Here's how the part is built. I have some questions about the finished solid (model axes, mm). A direction names the side the tool comes from. Give positions to 0.01 mm unless a question says otherwise; leave off trailing zeros. Write each loop counter-clockwise with the first axis right and the second up, starting at its lowest first coordinate (ties: lowest second). Pieces come first, ordered by that corner, then holes. Notation, with made-up numbers: (30.25, -38) -> (75.25, -38) arc R19 ccw to (75.25, -29) -> close; hole circle Ø11 at (-37.5, 55). An arc over 180 degrees is marked (long way). Return JSON: item names as keys, results as strings.
Solid Edge part; units mm, degrees
sketch "Sketch1" plane through (0, 0, 0) normal (0, -1, 0) x (1, 0, 0)
  line L0 (-10, -30.5) -> (0, -30.5)
  line L1 (0, 30.5) -> (0, -30.5)
  line L2 (0, 30.5) -> (-10, 30.5)
  line L3 (-10, 30.5) -> (-10, -30.5)
revolve "RevolvedProtrusion1" add sketch "Sketch1" angle 360 about axis through (0, 0, 54) along (0, 0, -1)
sketch "Sketch2" plane through (0, 0, 0) normal (1, 0, 0) x (0, 1, 0)
  circle A0 centre (0, 2) radius 10
extrude "Protrusion1" add sketch "Sketch2" along normal blind 150
sketch "Sketch3" plane through (0, 0, 0) normal (0, 0, 1) x (1, 0, 0)
  circle A0 centre (-25.6627, -96.6511) radius 5
  line L0 (-8.9463, -4.4682) -> (-32.9115, -94.7264)
  arc A1 (-32.9115, -94.7264) -> (-18.4138, -98.5758) centre (-25.6627, -96.6511) ccw
  line L1 (-18.4138, -98.5758) -> (5.5514, -8.3176)
  arc A2 (5.5514, -8.3176) -> (-8.9463, -4.4682) centre (0, 0) cw
  dimension "D1" = 32.9115
  dimension "D2" = 25.6627
extrude "Styrarm" add sketch "Sketch3" along normal mid plane 10
hole "Hole1" at (0, 0, 30.5) direction (0, 0, -1) diameter 10 end up to next
1. For pin 1 Ø5 at (x, z) = (46, 11.5) entering from -Y; pin 2 Ø1.5 at (x, z) = (67, 6) entering from +Y; pin 3 Ø10 at (y, z) = (-8, 2) entering from -X, each with a flat end and sliding along its axis, tell me the tip position at first contact or that it passes through.
Taken from the geometry:
{"pin 1": "stops at y = -7.14", "pin 2": "stops at y = 9.46", "pin 3": "stops at x = -11.21"}
2. Suppose I cut it at D-D, the plane x = 99. List the corners of the cut face in (y, z) for me.
Taken from the geometry:
{"outline": "circle Ø20 at (0, 2)"}
3. Suppose I cut it at B-B, the plane z = 2. List the corners of the cut face in (x, y) for me, and give its area (3 significant figures).
Taken from the geometry:
{"outline": "(-32.91, -94.73) arc R7.5 ccw to (-18.41, -98.58) -> (5.1, -10) -> (150, -10) -> (150, 10) -> (0, 10) arc R10 ccw to (-8.95, -4.47) -> close; hole circle Ø10 at (-25.66, -96.65); hole circle Ø10 at (0, 0)", "area": "4,450 mm²"}
4. Which directions (+Z, -Z, +X, -X, +Y, -Y) give clear straight access to the entire face, cutting with the end or side of a thin tool? Please do faces 1 (the face through (-9.54, 3, -0.43)), 2 (the face through (74, -10, 2)), 3 (the face through (-2, 5, -30.5)).
Taken from the geometry:
{"face 1": "none", "face 2": "+X", "face 3": "-Z, +X, -X, +Y, -Y"}
5. If I drill on line 1 (X direction, y = 0, z = 16); line 2 (X direction, y = 0, z = -4), over which ranges is the centre line in solid material (lowest first)? Write a range as [from, to].
Taken from the geometry:
{"line 1": "x = [-10, -5], [5, 10]", "line 2": "x = [-10, -5], [5, 150]"}
6. If we mould it in two halves opening along X, with no side actions, what happens to faces 4 (the face through (-6.6, -54.08, -0.07)), 5 (the face through (-4.88, 1.08, 0.43)), 6 (the face through (-22.975, -100.867, -0.07)), 7 (the face through (-12, -54, -5))? For each: released by +X, released by -X, zero draft, split by the parting line, or undercut.
Taken from the geometry:
{"face 4": "released by +X", "face 5": "undercut", "face 6": "undercut", "face 7": "zero draft"}
7. Suppose I cut it at C-C, the plane z = -17.5. List the corners of the cut face in (x, y) for me, and give its area (3 significant figures).
Taken from the geometry:
{"outline": "circle Ø20 at (0, 0); hole circle Ø10 at (0, 0)", "area": "236 mm²"}
8. Suppose I cut it at A-A, the plane y = 0. List the corners of the cut face in (x, z) for me.
Taken from the geometry:
{"outline": "(-10, -30.5) -> (-5, -30.5) -> (-5, 30.5) -> (-10, 30.5) -> close; (5, -30.5) -> (10, -30.5) -> (10, -8) -> (150, -8) -> (150, 12) -> (10, 12) -> (10, 30.5) -> (5, 30.5) -> close"}
